For this review, use the dimensioned drawing (mm, ordinates from the lowest corner) and the shaded views. A direction names the side the tool comes from. Give positions to 0.01 mm unless a question says otherwise; leave off trailing zeros. Loops run counter-clockwise (first coordinate to the right, second up) from the corner with the lowest first, then second, coordinate; pieces in that order, holes last. Notation, with made-up numbers: M -5,28 L 33,28 A29 ccw 33,48 Z; hole C 35.25,40.25 d11. An arc over 180 degrees is marked long. Use a Markdown table: item, result. Add a question column.
(1) Add section A-A, the plane x = 4.5. Give the boundary of the cut face in (y, z).
(2) Add section C-C, the plane y = 2.1. Give the boundary of the cut face in (x, z), then the cut area to 3 significant figures.
(3) Add section B-B, the plane z = 9. Give the boundary of the cut face in (x, y).
(4) Add section D-D, the plane x = 12. Give the boundary of the cut face in (y, z).
(5) For probe 1 along X at (y, z) = (1.45, 12.25); probe 2 along X at (y, z) = (2.2, 4); probe 3 along Z at (x, y) = (3, 1.65), list the stretches that pass through material, from the lowest coordinate up.
(6) For the marked faces 4 and 5, list the 3-axis set-ups (+Z, -Z, +X, -X, +Y, -Y) from which the entire face can be reached by the end or side of a thin tool; tool diameter is ignored.
(7) Insertion check: pin 1 Ø4 at (x, z) = (13, 8) entering from -Y. The pin has a flat end and moves straight along its axis. Give the tip position at first contact, or say it passes through.
(8) Draft analysis for pull direction X (two halves, no side actions). For the marked faces 1, 2 and 3, state which applies: pulls with the +X half, pulls with the -X half, needs draft (parallel to the pull), parting line crosses it, or undercut.
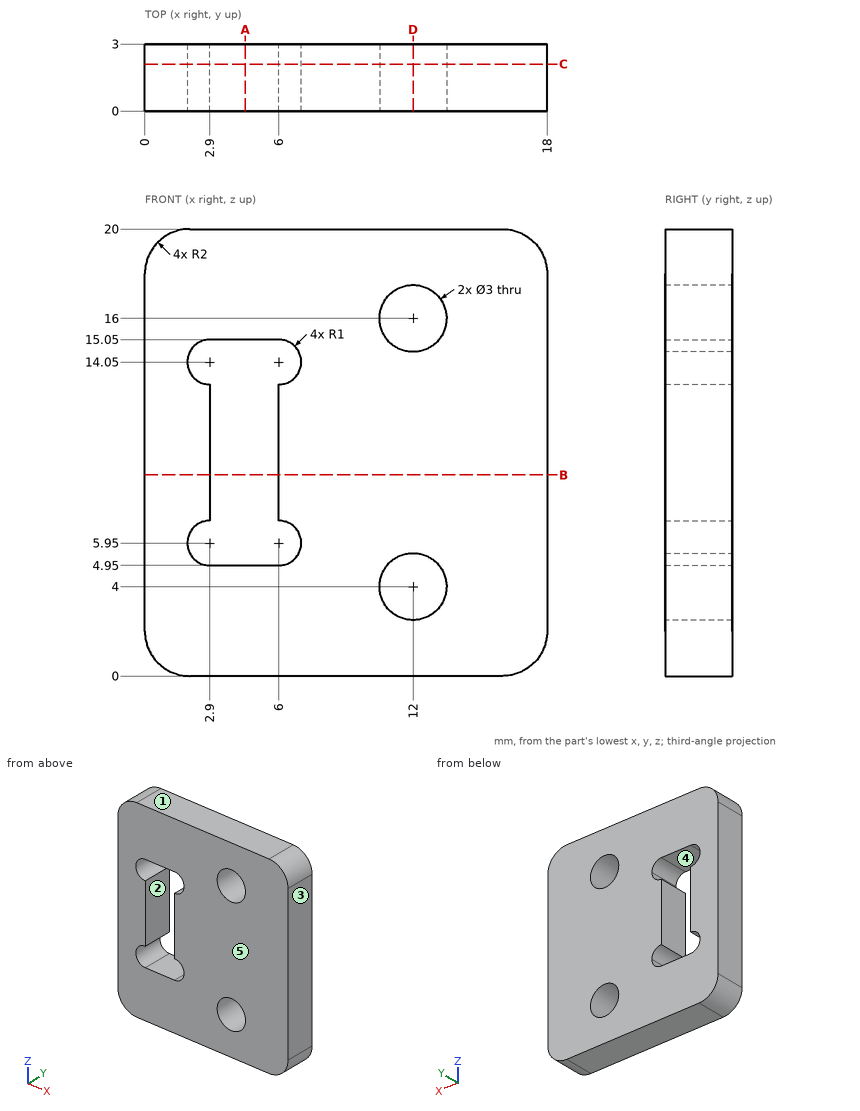
Established:
| question | item | result |
|---|---|---|
| 1 | outline | M 0,0 L 3,0 L 3,4.95 L 0,4.95 Z; M 0,15.05 L 3,15.05 L 3,20 L 0,20 Z |
| 2 | outline | M 0,2 A2 ccw 2,0 L 16,0 A2 ccw 18,2 L 18,18 A2 ccw 16,20 L 2,20 A2 ccw 0,18 Z; hole M 2.9,4.95 L 6,4.95 A1 ccw 6,6.95 L 6,13.05 A1 ccw 6,15.05 L 2.9,15.05 A1 ccw 2.9,13.05 L 2.9,6.95 A1 ccw Z; hole C 12,4 d3; hole C 12,16 d3 |
| 2 | area | 305 mm^2 |
| 3 | outline | M 0,0 L 2.9,0 L 2.9,3 L 0,3 Z; M 6,0 L 18,0 L 18,3 L 6,3 Z |
| 4 | outline | M 0,0 L 3,0 L 3,2.5 L 0,2.5 Z; M 0,5.5 L 3,5.5 L 3,14.5 L 0,14.5 Z; M 0,17.5 L 3,17.5 L 3,20 L 0,20 Z |
| 5 | probe 1 | 0 to 2.9, 6 to 18 |
| 5 | probe 2 | 0 to 10.5, 13.5 to 18 |
| 5 | probe 3 | 0 to 4.95, 15.05 to 20 |
| 6 | face 4 | +Y, -Y |
| 6 | face 5 | +Z, -Z, +X, -X, -Y |
| 7 | pin 1 | y = 0 |
| 8 | face 1 | needs draft |
| 8 | face 2 | undercut |
| 8 | face 3 | pulls with the +X half |
